Work out the finished part from the listing and answer in its coordinate system (mm). A direction names the side the tool comes from. Coordinates: 2 decimals unless noted, no trailing zeros. Loops run counter-clockwise (first coordinate to the right, second up) from the corner with the lowest first, then second, coordinate; pieces in that order, holes last. Notation, with made-up numbers: (78.5, -21) -> (106.5, -21) arc R9 ccw to (106.5, -13) -> close; hole circle Ø9 at (81, -9.75). An arc over 180 degrees is marked (long way). Use a Markdown table: item, result.
from build123d import *

# Parameters (mm, degrees)
ANGLE_IRON_2_X_2_X_0_125_1_DEPTH = 50
SKETCH4_R                        = 7.9375
CUT_EXTRUDE1_DEPTH               = 3.175
SKETCH3_R                        = 7.9375
CUT_EXTRUDE2_DEPTH               = 3.175


with BuildPart() as part:
    # Sketch1 → Angle iron 2 X 2 X 0.125(1) (new body)
    with BuildSketch(Plane(origin=(0, 0, 0), x_dir=(0, 0, -1), z_dir=(1, 0, 0))):
        with BuildLine():
            Line((0, 0), (0, 50.8))
            Line((0, 50.8), (0.00508, 50.8))
            ThreePointArc((0.00508, 50.8), (2.246551928, 49.871551928), (3.175, 47.63008))
            Line((3.175, 47.63008), (3.175, 7.9375))
            ThreePointArc((3.175, 7.9375), (4.569903955, 4.569903955), (7.9375, 3.175))
            Line((7.9375, 3.175), (47.63008, 3.175))
            ThreePointArc((47.63008, 3.175), (49.871551928, 2.246551928), (50.8, 0.00508))
            Line((50.8, 0.00508), (50.8, 0))
            Line((50.8, 0), (0, 0))
        make_face()
    extrude(amount=ANGLE_IRON_2_X_2_X_0_125_1_DEPTH)

    # Sketch4 → Cut-Extrude1 (cut)
    with BuildSketch(Plane(origin=(0, 3.175, 0), x_dir=(1, 0, 0), z_dir=(0, 1, 0))):
        with Locations(Location((25, 27.78379, 0), (0, 0, 270))):
            Circle(SKETCH4_R)
    extrude(amount=-CUT_EXTRUDE1_DEPTH, mode=Mode.SUBTRACT)

    # Sketch3 → Cut-Extrude2 (cut)
    with BuildSketch(Plane(origin=(0, 0, -3.175), x_dir=(-1, 0, 0), z_dir=(0, 0, -1))):
        with Locations(Location((-25, 34.9975, 0), (0, 0, 90))):
            Circle(SKETCH3_R)
    extrude(amount=-CUT_EXTRUDE2_DEPTH, mode=Mode.SUBTRACT)


solid = part.part
Q1. For faces 4 (the cylindrical face through (32.87, 1.61, -28.82)), 5 (the flat face through (25, 3.175, -36)), determine the directions among +Z, -Z, +X, -X, +Y, -Y from which every point of the face is accessible in a straight line to the end or side of a thin tool.
Solved:
| item | result |
|---|---|
| face 4 | +Y, -Y |
| face 5 | -Z, +X, -X, +Y |
Q2. Determine the mould class of faces 1 (the cylindrical face through (32.87, 33.96, -1.61)), 2 (the flat face through (0, 3, -14)), 3 (the flat face through (19, 0, -20)) for opening direction X: pulls with the +X half, pulls with the -X half, needs draft (parallel to the pull), parting line crosses it, or undercut.
Solved:
| item | result |
|---|---|
| face 1 | undercut |
| face 2 | pulls with the -X half |
| face 3 | needs draft |
Q3. Section B-B on y = 40.5 is taken. Determine the outline of the cut face in (x, z) (3 decimals), and give its area (3 significant figures).
Solved:
| item | result |
|---|---|
| outline | (0, -3.175) -> (19.279, -3.175) -> (19.279, 0) -> (0, 0) -> close; (30.721, -3.175) -> (50, -3.175) -> (50, 0) -> (30.721, 0) -> close |
| area | 122 mm² |
Q4. Given pin 1 Ø5 at (x, y) = (27, 20) entering from -Z (3 decimals); pin 2 Ø6 at (x, z) = (11, -43) entering from +Y (3 decimals); pin 3 Ø12.5 at (x, y) = (25, 35) entering from -Z, each flat-ended and moving along its own axis, determine where each tip first touches the part or whether it passes through.
Solved:
| item | result |
|---|---|
| pin 1 | z = -3.175 |
| pin 2 | y = 3.175 |
| pin 3 | through |
Q5. Section D-D on z = -32 is taken. Determine the outline of the cut face in (x, y) (3 decimals).
Solved:
| item | result |
|---|---|
| outline | (0, 0) -> (18.275, 0) -> (18.275, 3.175) -> (0, 3.175) -> close; (31.725, 0) -> (50, 0) -> (50, 3.175) -> (31.725, 3.175) -> close |
Q6. Section A-A on x = 25 is taken. State how many separate pieces and enclosed holes the cut face has, and give its area (3 significant figures).
Solved:
| item | result |
|---|---|
| separate pieces | 3 |
| enclosed holes | 0 |
| area | 212 mm² |
Q7. Consider line 1 (Y direction, x = 30, z = -18) (3 decimals); line 2 (Z direction, x = 24.5, y = 25.5) (3 decimals); line 3 (X direction, y = 2, z = -21). Determine where each line is inside the solid, lowest interval first. Write a range as [from, to].
Solved:
| item | result |
|---|---|
| line 1 | [0, 3.175] |
| line 2 | [-3.175, 0] |
| line 3 | [0, 20.88], [29.12, 50] |
